Model file for the job. Use its own axes, mm. Face numbers are marked on the shaded views. A direction names the side the tool comes from. Coordinates: 2 decimals unless noted, no trailing zeros. Order: outer loops, then holes, each group sorted by start corner. A loop starts at its lowest first (then second) coordinate and runs counter-clockwise, first axis right, second up. Notation, with made-up numbers: (65, 39) -> (82, 39) arc R25 ccw to (82, 65) -> close; hole circle Ø3 at (-24.75, 76.5). An arc over 180 degrees is marked (long way). Write item = value, one per line. Start each with the question number.
Q1. Wall check: line 1 (X direction, y = 145, z = 21.5); line 2 (X direction, y = 339, z = 28.5); line 3 (Z direction, x = -81.5, y = 154). Give the ranges that are in metal, low to high. Write a range as from..to.
Q2. Cut at D-D, the plane y = 98. List the corners of the cut face in (x, z), plus the area to 3 significant figures.
Q3. Cut at A-A, the plane y = 146. List the corners of the cut face in (x, z), plus the area to 3 significant figures.
Q4. 3-axis set-ups, long thin cutter, end or side, ignore diameter. For the marked faces 4 and 5: which of +Z, -Z, +X, -X, +Y, -Y reach the whole face in a straight line?
Q5. Cut at C-C, the plane x = -184. List the corners of the cut face in (y, z), plus the area to 3 significant figures.
Q6. Flat gauge pins, fed straight in: pin 1 (22.5 mm diameter, centred on y = 237.5, z = 18.5, fed in from +X); pin 2 (7.5 mm diameter, centred on y = 19.5, z = 18, fed in from -X); pin 3 (6 mm diameter, centred on x = -74.5, y = 252.5, fed in from +Z). Where does each tip first touch, or does it go through?
Q7. Cut at B-B, the plane x = -117. List the corners of the cut face in (y, z), plus the area to 4 significant figures.
Q8. Mould opens along X. For the marked faces 1, 2 and 3 say: +X half, -X half, draft (parallel to the pull), parting line (faces both ways), or undercut.
from build123d import *

# Parameters (mm, degrees)
F0_W      = 320
F0_H      = 430
F1_DEPTH  = 5
F2_W      = 35
F2_H      = 100
F3_DEPTH  = 5
F4_W      = 35
F4_H      = 100
F5_DEPTH  = 5
F7_DEPTH  = 5
F8_W      = 3
F8_H      = 70
F9_DEPTH  = 60
F10_W     = 3
F10_H     = 70
F11_DEPTH = 60
F12_W     = 5
F12_H     = 50
F13_DEPTH = 60
F14_W     = 5
F14_H     = 50
F15_DEPTH = 60
F16_R     = 10
F17_DEPTH = 120
F18_R     = 10.2640382995
F19_DEPTH = 240
F20_W     = 10
F20_H     = 15
F21_DEPTH = 30
F22_SIZE  = 14.99999
F23_W     = 10
F23_H     = 15
F24_DEPTH = 30
F25_SIZE  = 14.99999
F26_W     = 4
F26_H     = 45
F27_DEPTH = 45
F28_W     = 10
F28_H     = 60
F29_DEPTH = 40
F30_W     = 10
F30_H     = 60
F31_DEPTH = 40
F32_R     = 5
F33_DEPTH = 240
F34_R     = 5
F35_DEPTH = 240
F36_R     = 5
F37_DEPTH = 250
F38_R     = 5
F39_DEPTH = 300
F40_R     = 5
F41_DEPTH = 300
F42_R     = 5
F43_DEPTH = 300
F44_R     = 10
F45_DEPTH = 207.2868810425
F46_R     = 5
F47_DEPTH = 207.2868810425
F48_R     = 5
F49_DEPTH = 207.2868810425
F50_R     = 5
F51_DEPTH = 207.2868810425
F52_R     = 5
F53_DEPTH = 207.2868810425


# Not quite as in the source:
# - a fillet or chamfer is up to 0.001 mm smaller than in the source, because OpenCascade refuses the exact size


with BuildPart() as f1:
    # F0 (on Top) → F1 (new body)
    with BuildSketch(Plane.XY):
        with Locations((-47.2858810425, 185.3322760761)):
            Rectangle(F0_W, F0_H)
    extrude(amount=F1_DEPTH)

    # F2 (on face) → F3 (cut)
    with BuildSketch(Plane.XY.offset(5)):
        with Locations((-159.7858810425, 171.3026314974)):
            Rectangle(F2_W, F2_H)
    extrude(amount=-F3_DEPTH, mode=Mode.SUBTRACT)

    # F4 (on face) → F5 (cut)
    with BuildSketch(Plane(origin=(0, 0, 0), x_dir=(1, 0, 0), z_dir=(0, 0, -1))):
        with Locations((67.7159577608, -172.2117364407)):
            Rectangle(F4_W, F4_H)
    extrude(amount=-F5_DEPTH, mode=Mode.SUBTRACT)

    # F6 (on face) → F7 (cut)
    with BuildSketch(Plane.XY.offset(5)):
        Polygon((68.7382593751, 362.0384633541), (-166.2617406249, 362.0384633541), (-166.2617406249, 277.0384633541), (-65.0134384632, 277.0384633541), (-48.7617406249, 277.0384633541), (68.7382593751, 277.0384633541), align=None)
    extrude(amount=-F7_DEPTH, mode=Mode.SUBTRACT)

    # F8 (on face) → F9 (join)
    with BuildSketch(Plane.XY.offset(5)):
        with Locations((-205.7858810425, 172.665733695)):
            Rectangle(F8_W, F8_H)
    extrude(amount=F9_DEPTH)

    # F10 (on face) → F11 (join)
    with BuildSketch(Plane.XY.offset(5)):
        with Locations((111.2141189575, 176.3021534681)):
            Rectangle(F10_W, F10_H)
    extrude(amount=F11_DEPTH)

    # F12 (on face) → F13 (join)
    with BuildSketch(Plane.XY.offset(5)):
        with Locations((-204.7858810425, 323.5781848431)):
            Rectangle(F12_W, F12_H)
    extrude(amount=F13_DEPTH)

    # F14 (on face) → F15 (join)
    with BuildSketch(Plane.XY.offset(5)):
        with Locations((110.2141189575, 321.7600047588)):
            Rectangle(F14_W, F14_H)
    extrude(amount=F15_DEPTH)

    # F16 (on Right) → F17 (cut)
    with BuildSketch(Plane.YZ):
        with Locations((175.784942263, 45.0581042336)):
            Circle(F16_R)
    extrude(amount=F17_DEPTH, mode=Mode.SUBTRACT)

    # F18 (on Right) → F19 (cut)
    with BuildSketch(Plane.YZ):
        with Locations((176.2254685163, 45.2939495444)):
            Circle(F18_R)
    extrude(amount=-F19_DEPTH, mode=Mode.SUBTRACT)

    # F20 (on face) → F21 (join)
    with BuildSketch(Plane.XY.offset(5)):
        with Locations((107.7141189575, 18.3457679302)):
            Rectangle(F20_W, F20_H)
    extrude(amount=F21_DEPTH)

    # F22 (size 15 in the source; OpenCascade refuses exactly that, so slightly less here)
    f22_edges = [f1.edges().sort_by_distance(p)[0] for p in [
        (107.714119, 10.845768, 35),
    ]]
    chamfer(f22_edges, length=F22_SIZE)

    # F23 (on face) → F24 (join)
    with BuildSketch(Plane.XY.offset(5)):
        with Locations((-201.83388412, 19.7091826051)):
            Rectangle(F23_W, F23_H)
    extrude(amount=F24_DEPTH)

    # F25 (size 15 in the source; OpenCascade refuses exactly that, so slightly less here)
    f25_edges = [f1.edges().sort_by_distance(p)[0] for p in [
        (-201.833884, 12.209183, 35),
    ]]
    chamfer(f25_edges, length=F25_SIZE)

    # F26 (on face) → F27 (join)
    with BuildSketch(Plane.XY.offset(5)):
        with Locations((-43.3766950369, 227.4395442009)):
            Rectangle(F26_W, F26_H)
    extrude(amount=F27_DEPTH)

    # F28 (on face) → F29 (join)
    with BuildSketch(Plane.XY.offset(5)):
        with Locations((102.7141189575, 326.7600047588)):
            Rectangle(F28_W, F28_H)
    extrude(amount=F29_DEPTH)

    # F30 (on face) → F31 (join)
    with BuildSketch(Plane.XY.offset(5)):
        with Locations((-198.1973099709, 328.5773980618)):
            Rectangle(F30_W, F30_H)
    extrude(amount=F31_DEPTH)

    # F32 (on Right) → F33 (cut)
    with BuildSketch(Plane.YZ):
        with Locations((310.6648027897, 53.3718466759)):
            Circle(F32_R)
    extrude(amount=F33_DEPTH, mode=Mode.SUBTRACT)

    # F34 (on Right) → F35 (cut)
    with BuildSketch(Plane.YZ):
        with Locations((330.2825987339, 53.3718466759)):
            Circle(F34_R)
    extrude(amount=F35_DEPTH, mode=Mode.SUBTRACT)

    # F36 (on Right) → F37 (cut)
    with BuildSketch(Plane.YZ):
        with Locations((321.0507035255, 33.1770926714)):
            Circle(F36_R)
    extrude(amount=F37_DEPTH, mode=Mode.SUBTRACT)

    # F38 (on Right) → F39 (cut)
    with BuildSketch(Plane.YZ):
        with Locations((310.0878298283, 52.794855088)):
            Circle(F38_R)
    extrude(amount=-F39_DEPTH, mode=Mode.SUBTRACT)

    # F40 (on Right) → F41 (cut)
    with BuildSketch(Plane.YZ):
        with Locations((330.8595716953, 53.3718466759)):
            Circle(F40_R)
    extrude(amount=-F41_DEPTH, mode=Mode.SUBTRACT)

    # F42 (on Right) → F43 (cut)
    with BuildSketch(Plane.YZ):
        with Locations((321.627676487, 33.7540879846)):
            Circle(F42_R)
    extrude(amount=-F43_DEPTH, mode=Mode.SUBTRACT)

    # F44 (on Right) → F45 (cut, through all)
    with BuildSketch(Plane.YZ):
        with Locations((228.0015647411, 27.0902961493)):
            Circle(F44_R)
    extrude(amount=-F45_DEPTH, mode=Mode.SUBTRACT)

    # F46 (on Right) → F47 (cut, through all)
    with BuildSketch(Plane.YZ):
        with Locations((241.425678134, 41.8319888413)):
            Circle(F46_R)
    extrude(amount=-F47_DEPTH, mode=Mode.SUBTRACT)

    # F48 (on Right) → F49 (cut, through all)
    with BuildSketch(Plane.YZ):
        with Locations((240.8486753702, 12.9823405296)):
            Circle(F48_R)
    extrude(amount=-F49_DEPTH, mode=Mode.SUBTRACT)

    # F50 (on Right) → F51 (cut, through all)
    with BuildSketch(Plane.YZ):
        with Locations((213.0800783634, 41.6209772229)):
            Circle(F50_R)
    extrude(amount=-F51_DEPTH, mode=Mode.SUBTRACT)

    # F52 (on Right) → F53 (cut, through all)
    with BuildSketch(Plane.YZ):
        with Locations((211.7366492748, 12.104251422)):
            Circle(F52_R)
    extrude(amount=-F53_DEPTH, mode=Mode.SUBTRACT)


solid = f1.part
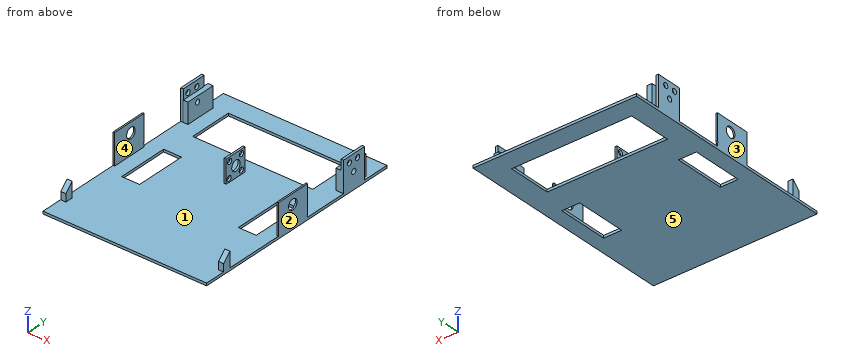
Here are the results:
q1.line_1 = -207.29..-204.29, 109.71..112.71
q1.line_2 = -207.29..-193.2, 97.71..112.71
q1.line_3 = 0..5
q2.outline = (-207.29, 0) -> (112.71, 0) -> (112.71, 5) -> (-207.29, 5) -> close
q2.area = 1,600 mm²
q3.outline = (-207.29, 0) -> (-177.29, 0) -> (-177.29, 5) -> (-204.29, 5) -> (-204.29, 65) -> (-207.29, 65) -> close; (-142.29, 0) -> (50.22, 0) -> (50.22, 5) -> (-142.29, 5) -> close; (85.22, 0) -> (112.71, 0) -> (112.71, 65) -> (109.71, 65) -> (109.71, 5) -> (85.22, 5) -> close
q3.area = 1,610 mm²
q4.face_4 = +Z
q4.face_5 = -Z, +X, -X, +Y, -Y
q5.outline = (-29.67, 0) -> (400.33, 0) -> (400.33, 5) -> (-29.67, 5) -> close
q5.area = 2,150 mm²
q6.pin_1 = -41.38
q6.pin_2 = -206.83
q6.pin_3 = 5
q7.outline = (-29.67, 0) -> (277.04, 0) -> (277.04, 5) -> (-29.67, 5) -> close; (362.04, 0) -> (400.33, 0) -> (400.33, 5) -> (362.04, 5) -> close
q7.area = 1,725 mm²
q8.face_1 = undercut
q8.face_2 = +X half
q8.face_3 = -X half
